```python
from build123d import *

# Parameters (mm, degrees)
CROQUIS1_R              = 4
SALIENTE_EXTRUIR1_DEPTH = 10
SALIENTE_EXTRUIR2_START = -10
SALIENTE_EXTRUIR2_DEPTH = 10
SALIENTE_EXTRUIR3_START = 12
CROQUIS3_R              = 6
SALIENTE_EXTRUIR3_DEPTH = 12
CAVIDAD2_START          = -12
CAVIDAD2_DEPTH          = 22


# Read off the part's stored shape, not the designer's step: Cavidad2
with BuildPart() as part:
    # Croquis1 → Saliente-Extruir1 (new body)
    with BuildSketch(Plane.XY):
        with BuildLine():
            ThreePointArc((2.63548484, 7.021696352), (3.092608138, 9.517786714), (2.0376941, 11.82572631))
            ThreePointArc((2.0376941, 11.82572631), (1.879375062, 11.85191754), (1.720719944, 11.875989343))
            ThreePointArc((1.720719944, 11.875989343), (0.003562929, 10.007620913), (-0.333938693, 7.492561975))
            ThreePointArc((-0.333938693, 7.492561975), (-1.171907523, 7.4078764), (-1.995097537, 7.2297708))
            ThreePointArc((-1.995097537, 7.2297708), (-3.092442124, 9.517840655), (-5.302458366, 10.764940096))
            ThreePointArc((-5.302458366, 10.764940096), (-5.445935977, 10.693071651), (-5.588439715, 10.61929101))
            ThreePointArc((-5.588439715, 10.61929101), (-5.879449513, 8.098429629), (-4.674179509, 5.86532573))
            ThreePointArc((-4.674179509, 5.86532573), (-5.3023336, 5.304267941), (-5.863620467, 4.676318533))
            ThreePointArc((-5.863620467, 4.676318533), (-8.096284603, 5.882402966), (-10.617251961, 5.592312652))
            ThreePointArc((-10.617251961, 5.592312652), (-10.691084574, 5.449835835), (-10.763005347, 5.306384448))
            ThreePointArc((-10.763005347, 5.306384448), (-9.516712076, 3.095913482), (-7.229042621, 1.997734411))
            ThreePointArc((-7.229042621, 1.997734411), (-7.407448462, 1.174609414), (-7.492439675, 0.336671529))
            ThreePointArc((-7.492439675, 0.336671529), (-10.007621547, 8.7279e-05), (-11.876616173, -1.716388149))
            ThreePointArc((-11.876616173, -1.716388149), (-11.85260224, -1.875052036), (-11.826468757, -2.033380616))
            ThreePointArc((-11.826468757, -2.033380616), (-9.518914087, -3.089136389), (-7.022657159, -2.632923552))
            ThreePointArc((-7.022657159, -2.632923552), (-6.683169782, -3.403709986), (-6.259401586, -4.131572556))
            ThreePointArc((-6.259401586, -4.131572556), (-8.096387206, -5.882261746), (-8.599516679, -8.369487015))
            ThreePointArc((-8.599516679, -8.369487015), (-8.486828706, -8.483733761), (-8.37262307, -8.596463397))
            ThreePointArc((-8.37262307, -8.596463397), (-5.885214453, -8.094241155), (-4.133855353, -6.257894208))
            ThreePointArc((-4.133855353, -6.257894208), (-3.406147397, -6.681927859), (-2.63548484, -7.021696352))
            ThreePointArc((-2.63548484, -7.021696352), (-3.092608138, -9.517786714), (-2.0376941, -11.82572631))
            ThreePointArc((-2.0376941, -11.82572631), (-1.879375062, -11.85191754), (-1.720719944, -11.875989343))
            ThreePointArc((-1.720719944, -11.875989343), (-0.003562929, -10.007620913), (0.333938693, -7.492561975))
            ThreePointArc((0.333938693, -7.492561975), (1.171907523, -7.4078764), (1.995097537, -7.2297708))
            ThreePointArc((1.995097537, -7.2297708), (3.092442124, -9.517840655), (5.302458366, -10.764940096))
            ThreePointArc((5.302458366, -10.764940096), (5.445935977, -10.693071651), (5.588439715, -10.61929101))
            ThreePointArc((5.588439715, -10.61929101), (5.879449513, -8.098429629), (4.674179509, -5.86532573))
            ThreePointArc((4.674179509, -5.86532573), (5.3023336, -5.304267941), (5.863620467, -4.676318533))
            ThreePointArc((5.863620467, -4.676318533), (8.096284603, -5.882402966), (10.617251961, -5.592312652))
            ThreePointArc((10.617251961, -5.592312652), (10.691084574, -5.449835835), (10.763005347, -5.306384448))
            ThreePointArc((10.763005347, -5.306384448), (9.516712076, -3.095913482), (7.229042621, -1.997734411))
            ThreePointArc((7.229042621, -1.997734411), (7.407448462, -1.174609414), (7.492439675, -0.336671529))
            ThreePointArc((7.492439675, -0.336671529), (10.007621547, -8.7279e-05), (11.876616173, 1.716388149))
            ThreePointArc((11.876616173, 1.716388149), (11.85260224, 1.875052036), (11.826468757, 2.033380616))
            ThreePointArc((11.826468757, 2.033380616), (9.518914087, 3.089136389), (7.022657159, 2.632923552))
            ThreePointArc((7.022657159, 2.632923552), (6.683169782, 3.403709986), (6.259401586, 4.131572556))
            ThreePointArc((6.259401586, 4.131572556), (8.096387206, 5.882261746), (8.599516679, 8.369487015))
            ThreePointArc((8.599516679, 8.369487015), (8.486828706, 8.483733761), (8.37262307, 8.596463397))
            ThreePointArc((8.37262307, 8.596463397), (5.885214453, 8.094241155), (4.133855353, 6.257894208))
            ThreePointArc((4.133855353, 6.257894208), (3.406147397, 6.681927859), (2.63548484, 7.021696352))
        make_face()
        Circle(CROQUIS1_R, mode=Mode.SUBTRACT)
    extrude(amount=SALIENTE_EXTRUIR1_DEPTH)

    # Croquis2 → Saliente-Extruir2 (add)
    with BuildSketch(Plane.XY.offset(10).offset(SALIENTE_EXTRUIR2_START)):
        with BuildLine():
            Line((3, 2.645751311), (3, -2.645751311))
            ThreePointArc((3, -2.645751311), (4, 0), (3, 2.645751311))
        make_face()
    extrude(amount=SALIENTE_EXTRUIR2_DEPTH)

    # Croquis3 → Saliente-Extruir3 (add)
    with BuildSketch(Plane(origin=(0, 0, 0), x_dir=(-1, 0, 0), z_dir=(0, 0, -1)).offset(SALIENTE_EXTRUIR3_START)):
        with Locations(Location((0, 0, 0), (0, 0, 180))):
            Circle(CROQUIS3_R)
        with BuildLine():
            Line((-3, -2.645751311), (-3, 2.645751311))
            ThreePointArc((-3, 2.645751311), (4, 0), (-3, -2.645751311))
        make_face(mode=Mode.SUBTRACT)
    extrude(amount=-SALIENTE_EXTRUIR3_DEPTH)

    # Cavidad2 outline → Cavidad2 (cut)
    with BuildSketch(Plane.XY.offset(CAVIDAD2_START)):
        with BuildLine():
            ThreePointArc((3.097941964, 2.72512385), (-4.112058036, 0), (3.097941964, -2.72512385))
            Line((3.097941964, -2.72512385), (3.097941964, 2.72512385))
        make_face()
        with BuildLine():
            Line((3, 2.645751311), (3, -2.645751311))
            ThreePointArc((3, -2.645751311), (-4, 0), (3, 2.645751311))
        make_face(mode=Mode.SUBTRACT)
    extrude(amount=CAVIDAD2_DEPTH, mode=Mode.SUBTRACT)


solid = part.part
```
Part model, mm, in its own coordinate system. Round coordinates to 2 decimals unless told otherwise and drop trailing zeros. Loops run counter-clockwise (first coordinate to the right, second up) from the corner with the lowest first, then second, coordinate; pieces in that order, holes last.
1. Flat gauge pins, fed straight in: pin 1 (1 mm diameter, centred on y = -6, z = -7, fed in from -X); pin 2 (12 mm diameter, centred on x = 8, z = 2.5, fed in from -Y); pin 3 (4 mm diameter, centred on x = 0.5, z = -8.5, fed in from +Y). Where does each tip first touch, or does it go through?
Solutions:
pin 1: stops at x = -2.4
pin 2: stops at y = -10.76
pin 3: stops at y = 6
2. Two-plate mould, pull along X, no slides. Class faces 1 (the face through (3.417, 6.677, 4.93)), 2 (the face through (-5.917, -8.112, 4.93)), 3 (the face through (5, -5, 0)): pulls with the +X half, pulls with the -X half, needs draft (parallel to the pull), parting line crosses it, or undercut.
Solutions:
face 1: undercut
face 2: undercut
face 3: needs draft
3. Drill centre lines: line 1 along X through (y, z) = (-8, 7); line 2 along Y through (x, z) = (-8, 3.25); line 3 along Y through (x, z) = (6.5, 1.5). Where is each one in solid material? Low to high.
Solutions:
line 1: x = -8.62 to -5.72, -3.01 to 0.39, 2.18 to 5.86
line 2: y = -8.62 to -5.72, -3 to 0.39, 2.18 to 5.86
line 3: y = -5.21 to 3.74, 4.26 to 8.37
4. Slice it at D-D (y = 9). Give the cut face in (x, z).
Solutions:
outline: (-5.95, 0) - (-2.68, 0) - (-2.68, 10) - (-5.95, 10) - close; (-0.32, 0) - (3.12, 0) - (3.12, 10) - (-0.32, 10) - close
5. Slice it at A-A (x = 0). Give the cut face in (y, z), and give its area (3 significant figures).
Solutions:
outline: (-10, 0) - (-6, 0) - (-6, -12) - (-4.12, -12) - (-4.12, 10) - (-10, 10) - close; (4.12, -12) - (6, -12) - (6, 0) - (10, 0) - (10, 10) - (4.12, 10) - close
area: 163 mm2
6. Slice it at C-C (z = -10). Give the cut face in (x, y).
Solutions:
outline: circle Ø12 at (0, 0); hole (3.1, -2.73) - (3.1, 2.73) arc R4.12 ccw (long way) to start
7. Slice it at B-B (y = 0). Give the cut face in (x, z), and give its area (3 significant figures).
Solutions:
outline: (-10.01, 0) - (-6, 0) - (-6, -12) - (-4.11, -12) - (-4.11, 10) - (-10.01, 10) - close; (3.1, -12) - (6, -12) - (6, 0) - (10.01, 0) - (10.01, 10) - (3.1, 10) - close
area: 186 mm2
